```python
from build123d import *
from OCP.BRepFilletAPI import BRepFilletAPI_MakeChamfer

# Parameters (mm, degrees)
RESSALTO_EXTRUS_O1_DEPTH = 5
RESSALTO_EXTRUS_O2_DEPTH = 29
CORTE_EXTRUS_O1_REACH    = 89.714
RESSALTO_EXTRUS_O3_DEPTH = 5
ESBO_O5_W                = 13.5
ESBO_O5_H                = 17.397720337
RESSALTO_EXTRUS_O4_DEPTH = 8
RESSALTO_EXTRUS_O5_DEPTH = 20
ESBO_O7_W                = 11.5
ESBO_O7_H                = 13
CORTE_EXTRUS_O2_DEPTH    = 20
RESSALTO_EXTRUS_O6_DEPTH = 20
ESBO_O9_W                = 12
ESBO_O9_H                = 15
CORTE_EXTRUS_O3_DEPTH    = 20
ESBO_O11_W               = 6
ESBO_O11_H               = 39.4
RESSALTO_EXTRUS_O7_DEPTH = 5
ESBO_O12_W               = 6
ESBO_O12_H               = 41.397720337
RESSALTO_EXTRUS_O8_DEPTH = 5
CHANFRO1_SIZE            = 5
CHANFRO1_SIZE_2          = 6
RESSALTO_EXTRUS_O9_START = -5.7
RESSALTO_EXTRUS_O9_DEPTH = 6
ESBO_O14_R               = 1.6
CORTE_EXTRUS_O4_DEPTH    = 6


with BuildPart() as part:
    # Esboço1 → Ressalto-extrusão1 (new body)
    with BuildSketch(Plane.XY):
        Polygon((0, 0), (0, 58.4), (20, 58.4), (20, 25.2), (29, 17.52), (29, 0), align=None)
    extrude(amount=RESSALTO_EXTRUS_O1_DEPTH)

    # Esboço2 → Ressalto-extrusão2 (add)
    with BuildSketch(Plane.ZY):
        with BuildLine():
            Line((0, 0), (5, 0))
            ThreePointArc((5, 0), (2.871117767, -9.744454942), (-6.101940178, -14.1))
            Line((-6.101940178, -14.1), (-39.10228157, -14.1))
            ThreePointArc((-39.10228157, -14.1), (-48.076340899, -9.74361665), (-50.204561234, 0.002279663))
            Line((-50.204561234, 0.002279663), (-50.204561234, 61.4))
            Line((-50.204561234, 61.4), (-45.204561234, 61.4))
            Line((-45.204561234, 61.4), (-45.204561234, 9.002278982))
            ThreePointArc((-45.204561234, 9.002278982), (-40.78120589, -1.676645138), (-30.10228157, -6.1))
            Line((-30.10228157, -6.1), (-6.102283186, -6.1))
            ThreePointArc((-6.102283186, -6.1), (-1.788124517, -4.313489814), (0, 0))
        make_face()
    extrude(amount=-RESSALTO_EXTRUS_O2_DEPTH)

    # Esboço3 → Corte-extrusão1 (cut, up to next)
    with BuildSketch(Plane(origin=(0, 0, -50.204561234), x_dir=(-1, 0, 0), z_dir=(0, 0, -1)), mode=Mode.PRIVATE) as corte_extrus_o1_sk1:
        Polygon((-29, 17.52), (-20, 25.201139832), (-20, 61.4), (-29, 61.4), align=None)
    corte_extrus_o1_tool1 = extrude(corte_extrus_o1_sk1.sketch, amount=-CORTE_EXTRUS_O1_REACH, mode=Mode.PRIVATE) & part.part
    add(corte_extrus_o1_tool1.solids().sort_by_distance((24.64388, 41.318887, -50.204561))[0], mode=Mode.SUBTRACT)

    # Esboço4 → Ressalto-extrusão3 (add)
    with BuildSketch(Plane(origin=(0, 0, -50.204561234), x_dir=(-1, 0, 0), z_dir=(0, 0, -1))):
        Polygon((0, 34.002279663), (9.999992371, 44.002279663), (18.699996948, 44.002279663), (18.699996948, 61.4), (0, 61.4), align=None)
    extrude(amount=-RESSALTO_EXTRUS_O3_DEPTH)

    # Esboço5 → Ressalto-extrusão4 (add)
    with BuildSketch(Plane.XY.offset(-45.204561234)):
        with Locations((-11.949996948, 52.701139832)):
            Rectangle(ESBO_O5_W, ESBO_O5_H)
    extrude(amount=RESSALTO_EXTRUS_O4_DEPTH)

    # Esboço6 → Ressalto-extrusão5 (add)
    with BuildSketch(Plane(origin=(20, 0, 0), x_dir=(0, 0, -1), z_dir=(1, 0, 0))):
        Polygon((50.204561234, 58.4), (65.204561234, 58.4), (65.204561234, 51.4), (50.204561234, 41.4), align=None)
    extrude(amount=-RESSALTO_EXTRUS_O5_DEPTH)

    # Esboço7 → Corte-extrusão2 (cut)
    with BuildSketch(Plane(origin=(0, 0, -50.204561234), x_dir=(-1, 0, 0), z_dir=(0, 0, -1))):
        with Locations((-10.25, 47.9)):
            Rectangle(ESBO_O7_W, ESBO_O7_H)
    extrude(amount=CORTE_EXTRUS_O2_DEPTH, mode=Mode.SUBTRACT)

    # Esboço8 → Ressalto-extrusão6 (add)
    with BuildSketch(Plane(origin=(20, 0, 0), x_dir=(0, 0, -1), z_dir=(1, 0, 0))):
        Polygon((-5, 58.4), (-19.999999523, 58.4), (-19.999999523, 49.4), (-5, 39.4), align=None)
    extrude(amount=-RESSALTO_EXTRUS_O6_DEPTH)

    # Esboço9 → Corte-extrusão3 (cut)
    with BuildSketch(Plane.XY.offset(5)):
        with Locations((10, 46.9)):
            Rectangle(ESBO_O9_W, ESBO_O9_H)
    extrude(amount=CORTE_EXTRUS_O3_DEPTH, mode=Mode.SUBTRACT)

    # Esboço11 → Ressalto-extrusão7 (add)
    with BuildSketch(Plane.XY.offset(5)):
        with Locations((10, 19.7)):
            Rectangle(ESBO_O11_W, ESBO_O11_H)
    extrude(amount=RESSALTO_EXTRUS_O7_DEPTH)

    # Esboço12 → Ressalto-extrusão8 (add)
    with BuildSketch(Plane(origin=(0, 0, -50.204561234), x_dir=(-1, 0, 0), z_dir=(0, 0, -1))):
        with Locations((-10.25, 20.701139832)):
            Rectangle(ESBO_O12_W, ESBO_O12_H)
    extrude(amount=RESSALTO_EXTRUS_O8_DEPTH)

    # Chanfro1
    chanfro1_edges_1 = [part.edges().sort_by_distance(p)[0] for p in [
        (10, 0, 10),
    ]]
    chanfro1_side_1 = [part.faces().sort_by_distance(p)[0] for p in [
        (10, 0, 9.9),
    ]]
    chanfro1_edges_2 = [part.edges().sort_by_distance(p)[0] for p in [
        (10, 39.4, 10),
    ]]
    chanfro1_side_2 = [part.faces().sort_by_distance(p)[0] for p in [
        (10, 39.4, 9.9),
    ]]
    chanfro1_edges_3 = [part.edges().sort_by_distance(p)[0] for p in [
        (10.25, 0.002279663, -55.204561234),
    ]]
    chanfro1_side_3 = [part.faces().sort_by_distance(p)[0] for p in [
        (10.25, 0.002279663, -55.104561234),
    ]]
    chanfro1_edges_4 = [part.edges().sort_by_distance(p)[0] for p in [
        (10.25, 41.4, -55.204561234),
    ]]
    chanfro1_side_4 = [part.faces().sort_by_distance(p)[0] for p in [
        (10.25, 41.4, -55.104561234),
    ]]
    chanfro1 = BRepFilletAPI_MakeChamfer(part.part.solid().wrapped)
    for e in chanfro1_edges_1:
        chanfro1.Add(CHANFRO1_SIZE - 0.0001, CHANFRO1_SIZE_2 - 0.0001, e.wrapped, chanfro1_side_1[0].wrapped)
    for e in chanfro1_edges_2:
        chanfro1.Add(CHANFRO1_SIZE - 0.0001, CHANFRO1_SIZE_2 - 0.0001, e.wrapped, chanfro1_side_2[0].wrapped)
    for e in chanfro1_edges_3:
        chanfro1.Add(CHANFRO1_SIZE - 0.0001, CHANFRO1_SIZE_2 - 0.0001, e.wrapped, chanfro1_side_3[0].wrapped)
    for e in chanfro1_edges_4:
        chanfro1.Add(CHANFRO1_SIZE - 0.0001, CHANFRO1_SIZE_2 - 0.0001, e.wrapped, chanfro1_side_4[0].wrapped)
    add(Compound.cast(chanfro1.Shape()), mode=Mode.REPLACE)  # a hair under: the kernel refuses the full size

    # Esboço13 → Ressalto-extrusão9 (add)
    with BuildSketch(Plane(origin=(0, 61.4, 0), x_dir=(1, 0, 0), z_dir=(0, 1, 0)).offset(RESSALTO_EXTRUS_O9_START)):
        Polygon((-18.699996948, 50.204561234), (-18.699996948, 53.204561234), (0, 59.204561234), (0, 50.204561234), align=None)
    extrude(amount=-RESSALTO_EXTRUS_O9_DEPTH)

    # Esboço14 → Corte-extrusão4 (cut)
    with BuildSketch(Plane(origin=(0, 58.4, 0), x_dir=(1, 0, 0), z_dir=(0, 1, 0))):
        with Locations(Location((10.3, 57.704561234, 0), (0, 0, 270))):
            Circle(ESBO_O14_R)
        with Locations(Location((10, -12.499999523, 0), (0, 0, 270))):
            Circle(ESBO_O14_R)
    extrude(amount=-CORTE_EXTRUS_O4_DEPTH, mode=Mode.SUBTRACT)


solid = part.part
```
The model under review builds one solid part; all positions refer to its coordinate system, in mm. A direction names the side the tool comes from. Round coordinates to 2 decimals unless told otherwise and drop trailing zeros. Order: outer loops, then holes, each group sorted by start corner. A loop starts at its lowest first (then second) coordinate and runs counter-clockwise, first axis right, second up.
Item 1: Draft analysis for pull direction Y (two halves, no side actions). For faces 5 (the flat face through (10.29, 38.36, -52.74)), 6 (the flat face through (24.56, 21.31, -47.74)), 7 (the flat face through (-12, 53, -37.205)), state which applies: released by +Y, released by -Y, zero draft, split by the parting line, or undercut.
Working result:
face 5: undercut
face 6: released by +Y
face 7: zero draft
Item 2: Add section C-C, the plane y = 23. State the section outline as (x, z) points.
Working result:
outline: (0, -50.2) - (7.25, -50.2) - (7.25, -55.2) - (13.25, -55.2) - (13.25, -50.2) - (22.58, -50.2) - (22.58, -45.2) - (0, -45.2) - close; (0, 0) - (22.58, 0) - (22.58, 5) - (13, 5) - (13, 10) - (7, 10) - (7, 5) - (0, 5) - close
Item 3: Add section D-D, the plane z = -22. State the section outline as (x, y) points.
Working result:
outline: (0, -14.1) - (29, -14.1) - (29, -6.1) - (0, -6.1) - close
Item 4: Machinability: for faces 1 (the flat face through (-7, 49.7, -54)), 2 (the flat face through (10, 20, 10)), 3 (the flat face through (13.25, 20, -53)), 4 (the flat face through (10, 21, -55.205)), which of the approach directions +Z, -Z, +X, -X, +Y, -Y give a long, thin tool a straight path to every point of the face, cutting with its end or side? Answer none if there is none.
Working result:
face 1: -Z, -X, -Y
face 2: +Z, +X, -X, -Y
face 3: -Z, +X
face 4: -Z, +X, -X, -Y
Item 5: To check wall thickness, follow probe 1 along Z at (x, y) = (13, 46); probe 2 along X at (y, z) = (56.85, 12.5); probe 3 along Y at (x, z) = (23, -13.5). State the ranges of each line that lie inside material, in increasing order.
Working result:
probe 1: z = -50.2 to -45.2, 0 to 5
probe 2: x = 0 to 8.4, 11.6 to 20
probe 3: y = -14.1 to -6.1
Item 6: Add section A-A, the plane z = 12.5. State the section outline as (x, y) points, and give its area (3 significant figures).
Working result:
outline: (0, 44.4) - (4, 44.4) - (4, 54.4) - (8.4, 54.4) - (8.4, 58.4) - (0, 58.4) - close; (11.6, 54.4) - (16, 54.4) - (16, 44.4) - (20, 44.4) - (20, 58.4) - (11.6, 58.4) - close
area: 147 mm2
Item 7: For pin 1 (2.5 mm diameter, centred on y = 16.5, z = -53.5, fed in from +X); pin 2 (10 mm diameter, centred on x = 20.5, y = 8, fed in from +Z); pin 3 (10 mm diameter, centred on x = -12.5, z = -55.5, fed in from -Y); pin 4 (4 mm diameter, centred on x = -2.5, y = 20, fed in from -Z), all flat-tipped, find the tip position at first contact; note any pin that passes through.
Working result:
pin 1: stops at x = 13.25
pin 2: stops at z = 5
pin 3: stops at y = 49.7
pin 4: passes through
Item 8: Add section B-B, the plane x = 1.5. State the section outline as (y, z) points.
Working result:
outline: (-14.1, -39.1) arc R11.42 ccw to (0, -50.2) - (41.4, -50.2) - (51.4, -65.2) - (58.4, -65.2) - (58.4, -50.2) - (61.4, -50.2) - (61.4, -45.2) - (9, -45.2) arc R15.1 cw to (-6.1, -30.1) - (-6.1, -6.1) arc R6.1 cw to (0, 0) - (58.4, 0) - (58.4, 20) - (49.4, 20) - (39.4, 5) - (0, 5) arc R11.42 ccw to (-14.1, -6.1) - close
